from build123d import *

# Parameters (mm, degrees)
SKETCH1_W           = 40
SKETCH1_H           = 40
SKETCH1_R           = 12.5
SKETCH1_R_2         = 1
BOSS_EXTRUDE2_DEPTH = 1
SKETCH2_W           = 40
SKETCH2_H           = 1
BOSS_EXTRUDE3_DEPTH = 15
SKETCH3_R           = 1.5
CUT_EXTRUDE1_DEPTH  = 2


with BuildPart() as part:
    # Sketch1 → Boss-Extrude2 (new body)
    with BuildSketch(Plane.XY):
        Rectangle(SKETCH1_W, SKETCH1_H)
        Circle(SKETCH1_R, mode=Mode.SUBTRACT)
        with Locations((0, 15)):
            Circle(SKETCH1_R_2, mode=Mode.SUBTRACT)
        with Locations((7.5, 12.990381057)):
            Circle(SKETCH1_R_2, mode=Mode.SUBTRACT)
        with Locations((12.990381057, 7.5)):
            Circle(SKETCH1_R_2, mode=Mode.SUBTRACT)
        with Locations((15, 0)):
            Circle(SKETCH1_R_2, mode=Mode.SUBTRACT)
        with Locations((12.990381057, -7.5)):
            Circle(SKETCH1_R_2, mode=Mode.SUBTRACT)
        with Locations((7.5, -12.990381057)):
            Circle(SKETCH1_R_2, mode=Mode.SUBTRACT)
        with Locations((0, -15)):
            Circle(SKETCH1_R_2, mode=Mode.SUBTRACT)
        with Locations((-7.5, -12.990381057)):
            Circle(SKETCH1_R_2, mode=Mode.SUBTRACT)
        with Locations((-12.990381057, -7.5)):
            Circle(SKETCH1_R_2, mode=Mode.SUBTRACT)
        with Locations((-15, 0)):
            Circle(SKETCH1_R_2, mode=Mode.SUBTRACT)
        with Locations((-12.990381057, 7.5)):
            Circle(SKETCH1_R_2, mode=Mode.SUBTRACT)
        with Locations((-7.5, 12.990381057)):
            Circle(SKETCH1_R_2, mode=Mode.SUBTRACT)
    extrude(amount=BOSS_EXTRUDE2_DEPTH)

    # Sketch2 → Boss-Extrude3 (add)
    with BuildSketch(Plane.XY.offset(1)):
        with Locations((0, -20.5)):
            Rectangle(SKETCH2_W, SKETCH2_H)
    extrude(amount=-BOSS_EXTRUDE3_DEPTH)

    # Sketch3 → Cut-Extrude1 (cut, through all)
    with BuildSketch(Plane(origin=(0, -20, 0), x_dir=(1, 0, 0), z_dir=(0, 1, 0))):
        with Locations((-15, 7)):
            Circle(SKETCH3_R)
        with Locations((15, 7)):
            Circle(SKETCH3_R)
    extrude(amount=-CUT_EXTRUDE1_DEPTH, mode=Mode.SUBTRACT)


solid = part.part
Geometry: final body of the model. Coordinates: model frame, mm. Give positions to 0.01 mm unless a question says otherwise; leave off trailing zeros. Loops run counter-clockwise (first coordinate to the right, second up) from the corner with the lowest first, then second, coordinate; pieces in that order, holes last. Notation, with made-up numbers: (89, 56) -> (140, 56) arc R29 ccw to (140, 78) -> close; hole circle Ø1 at (68.25, 7.25). An arc over 180 degrees is marked (long way). Put each result on its own line as item: value.
1. Pin query (flat end, axial travel): P1, Ø1.2, axis at x = 12.99, y = 7.5, coming from the +Z side; P2, Ø2.5, axis at x = -7.5, y = 12.99, coming from the -Z side; P3, Ø1, axis at x = -9, z = -6, coming from the +Y side. Return the tip coordinate at first contact, or that it passes through.
Taken from the geometry:
P1: passes through
P2: stops at z = 0
P3: stops at y = -20
2. Pull-direction query (Z, two-part tool) for faces 1 (the flat face through (-0.3, -20.5, -14)), 2 (the cylindrical face through (13.8, -20.5, -6.1)), 3 (the flat face through (0, -20, -7)); classes: released by +Z, released by -Z, zero draft, split by the parting line, or undercut.
Taken from the geometry:
face 1: released by -Z
face 2: undercut
face 3: zero draft
3. Cut plane C-C (z = -7). Return the cut outline in (x, y), plus the area to 3 significant figures.
Taken from the geometry:
outline: (-20, -21) -> (-16.5, -21) -> (-16.5, -20) -> (-20, -20) -> close; (-13.5, -21) -> (13.5, -21) -> (13.5, -20) -> (-13.5, -20) -> close; (16.5, -21) -> (20, -21) -> (20, -20) -> (16.5, -20) -> close
area: 34.0 mm2
4. Cut plane D-D (y = 15). Return the cut outline in (x, z), plus the area to 3 significant figures.
Taken from the geometry:
outline: (-20, 0) -> (-1, 0) -> (-1, 1) -> (-20, 1) -> close; (1, 0) -> (20, 0) -> (20, 1) -> (1, 1) -> close
area: 38.0 mm2
5. Cut plane B-B (x = -15). Return the cut outline in (y, z).
Taken from the geometry:
outline: (-21, -14) -> (-20, -14) -> (-20, -8.5) -> (-21, -8.5) -> close; (-21, -5.5) -> (-20, -5.5) -> (-20, 0) -> (-1, 0) -> (-1, 1) -> (-21, 1) -> close; (1, 0) -> (20, 0) -> (20, 1) -> (1, 1) -> close
6. Cut plane A-A (y = 7.5). Return the cut outline in (x, z).
Taken from the geometry:
outline: (-20, 0) -> (-13.99, 0) -> (-13.99, 1) -> (-20, 1) -> close; (-11.99, 0) -> (-10, 0) -> (-10, 1) -> (-11.99, 1) -> close; (10, 0) -> (11.99, 0) -> (11.99, 1) -> (10, 1) -> close; (13.99, 0) -> (20, 0) -> (20, 1) -> (13.99, 1) -> close
7. Ray query, line 1 along Y through (x, z) = (7.5, 0.35); line 2 along Z through (x, y) = (12, 18); line 3 along Y through (x, z) = (1.5, -0.75). Return the intervals inside material, ascending. Write a range as [from, to].
Taken from the geometry:
line 1: y = [-21, -13.99], [-11.99, -10], [10, 11.99], [13.99, 20]
line 2: z = [0, 1]
line 3: y = [-21, -20]
